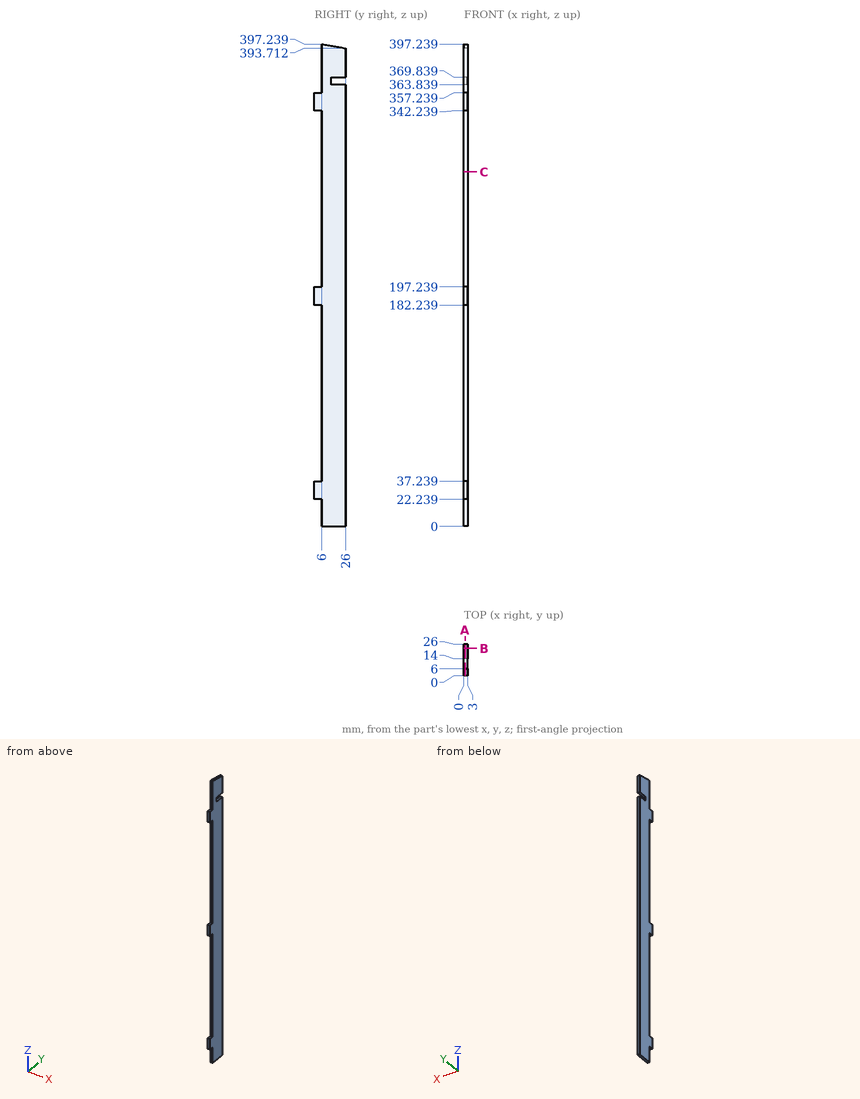
Could you check a few things on this drawing? It's one solid part, dimensions in mm from its lowest x, y, z. Coordinates: 2 decimals unless noted, no trailing zeros. Order: outer loops, then holes, each group sorted by start corner. A loop starts at its lowest first (then second) coordinate and runs counter-clockwise, first axis right, second up.
1) Imagine slicing it at B-B on y = 22.75. List the corners of the cut face in (x, z) for me (1 decimal).
2) I need wall thicknesses on line 1 (Z direction, x = 2, y = 2.75); line 2 (Z direction, x = 1.7, y = 14.5); line 3 (Z direction, x = 0.2, y = 17.5). Which ranges of each line are inside material? Lowest first, please.
3) Imagine slicing it at A-A on x = 1. List the corners of the cut face in (y, z) for me, and give its area (3 significant figures).
4) Will these pins go through, and if not, where does the flat tip stop? pin 1 (3 mm diameter, centred on y = 3, z = 333, fed in from -X); pin 2 (1.5 mm diameter, centred on x = 2.5, y = 3.5, fed in from -Z); pin 3 (0.9 mm diameter, centred on x = 2, y = 2, fed in from +Z); pin 4 (1.5 mm diameter, centred on x = 1.5, z = 111, fed in from -Y).
5) Imagine slicing it at C-C on z = 292. List the corners of the cut face in (x, y) for me.
Response values:
1. outline: (0, 0) - (3, 0) - (3, 363.8) - (0, 363.8) - close; (0, 369.8) - (3, 369.8) - (3, 394.3) - (0, 394.3) - close
2. line 1: z = 22.24 to 37.24, 182.24 to 197.24, 342.24 to 357.24
2. line 2: z = 0 to 363.84, 369.84 to 395.74
2. line 3: z = 0 to 363.84, 369.84 to 395.21
3. outline: (0, 22.24) - (6, 22.24) - (6, 0) - (26, 0) - (26, 363.84) - (14, 363.84) - (14, 369.84) - (26, 369.84) - (26, 393.71) - (6, 397.24) - (6, 357.24) - (0, 357.24) - (0, 342.24) - (6, 342.24) - (6, 197.24) - (0, 197.24) - (0, 182.24) - (6, 182.24) - (6, 37.24) - (0, 37.24) - close
3. area: 8,110 mm2
4. pin 1: passes through
4. pin 2: stops at z = 22.24
4. pin 3: stops at z = 357.24
4. pin 4: stops at y = 6
5. outline: (0, 6) - (3, 6) - (3, 26) - (0, 26) - close
